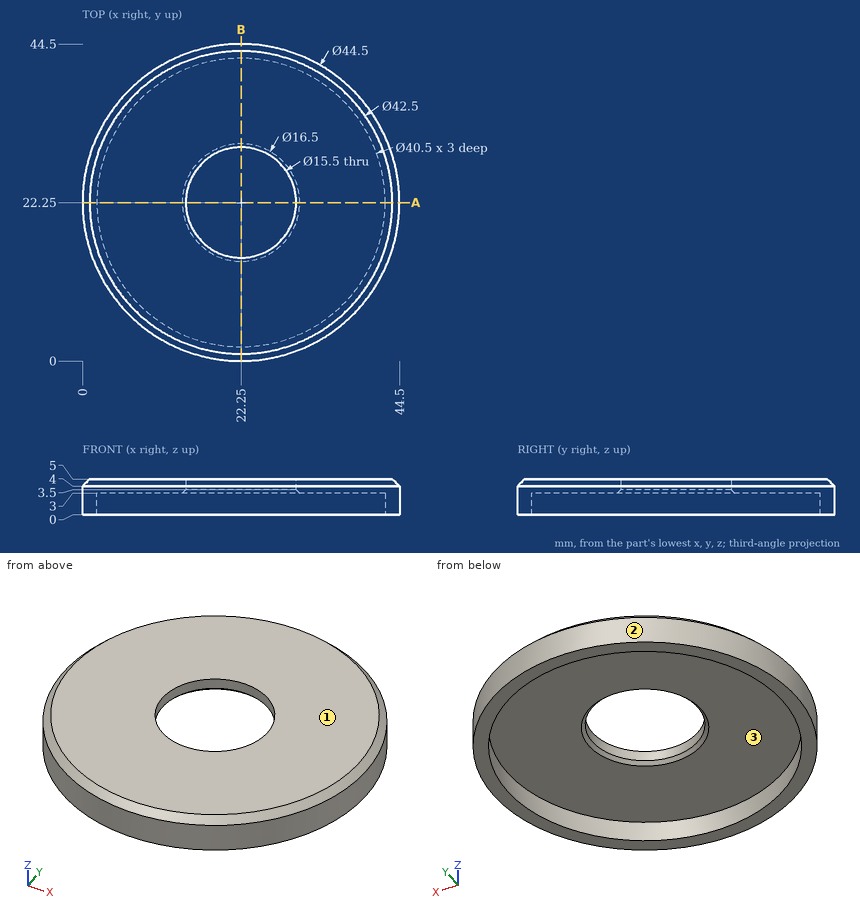
Can you work these out from the drawing? Everything is in mm from the part's minimum corner. Coordinates: 2 decimals unless noted, no trailing zeros. Write each loop counter-clockwise with the first axis right and the second up, starting at its lowest first coordinate (ties: lowest second). Pieces come first, ordered by that corner, then holes. Notation, with made-up numbers: (72.25, 30) - (93.25, 30) arc R8 ccw to (93.25, 35) - close; hole circle Ø4 at (48.5, 64.5). An arc over 180 degrees is marked (long way). Use a Markdown table: item, result.
Q1. Imagine slicing it at A-A (y = 22.25). List the corners of the cut face in (x, z) for me, and give its area (4 significant figures).
Geometry check:
| item | result |
|---|---|
| outline | (0, 0) - (2, 0) - (2, 3) - (14, 3) - (14.5, 3.5) - (14.5, 5) - (1, 5) - (0, 4) - close; (30, 3.5) - (30.5, 3) - (42.5, 3) - (42.5, 0) - (44.5, 0) - (44.5, 4) - (43.5, 5) - (30, 5) - close |
| area | 68.75 mm2 |
Q2. Please list where these lines run through material, in increasing order: L1, parallel to Y at x = 22.25, z = 4; L2, parallel to Y at x = 22.25, z = 1.9; L3, parallel to Z at x = 8, y = 8.
Geometry check:
| item | result |
|---|---|
| L1 | y = 0 to 14.5, 30 to 44.5 |
| L2 | y = 0 to 2, 42.5 to 44.5 |
| L3 | z = 3 to 5 |
Q3. Thinking about a two-plate mould opening in Y: for the marked faces 1, 2 and 3, which applies, +Y half, -Y half, draft (parallel to the pull), parting line (faces both ways), or undercut?
Geometry check:
| item | result |
|---|---|
| face 1 | draft |
| face 2 | parting line |
| face 3 | undercut |
Q4. I'm going to push flat-ended pins straight in: pin 1 Ø20 at (x, y) = (22.25, 22.25) entering from -Z; pin 2 Ø1 at (x, z) = (32, 1.5) entering from +Y; pin 3 Ø3 at (x, z) = (24, 3.5) entering from -Y. Where does each tip first touch, or does it pass through?
Geometry check:
| item | result |
|---|---|
| pin 1 | stops at z = 3 |
| pin 2 | stops at y = 42.49 |
| pin 3 | stops at y = 0 |
